Check sheet for the modelled part. Datum: model origin and axes. Units: mm. A direction names the side the tool comes from. Round coordinates to 2 decimals unless told otherwise and drop trailing zeros. Write each loop counter-clockwise with the first axis right and the second up, starting at its lowest first coordinate (ties: lowest second). Pieces come first, ordered by that corner, then holes. Notation, with made-up numbers: M -38.5,56 L 17.5,56 A27 ccw 17.5,83 Z; hole C -29,59 d1. An arc over 180 degrees is marked long. One line per item, written item: value.
from build123d import *

# Parameters (mm, degrees)
ESBO_O1_W                = 92
ESBO_O1_H                = 82
RESSALTO_EXTRUS_O1_DEPTH = 1.5
ESBO_O2_W                = 19
ESBO_O2_H                = 65
RESSALTO_EXTRUS_O2_DEPTH = 8.5
ESBO_O3_W                = 3
ESBO_O3_H                = 9
RESSALTO_EXTRUS_O3_DEPTH = 30.9
ESBO_O4_R                = 1.5
CORTE_EXTRUS_O1_DEPTH    = 3
ESBO_O5_R                = 1.5
CORTE_EXTRUS_O2_DEPTH    = 1.5
FILETE1_R                = 5
FILETE2_R                = 1


with BuildPart() as part:
    # Esboço1 → Ressalto-extrusão1 (new body)
    with BuildSketch(Plane(origin=(0, 0, 0), x_dir=(1, 0, 0), z_dir=(0, 1, 0))):
        Rectangle(ESBO_O1_W, ESBO_O1_H)
    extrude(amount=RESSALTO_EXTRUS_O1_DEPTH)

    # Esboço2 → Ressalto-extrusão2 (add)
    with BuildSketch(Plane(origin=(0, 1.5, 0), x_dir=(1, 0, 0), z_dir=(0, 1, 0))):
        with Locations((-33.5, -1.5)):
            Rectangle(ESBO_O2_W, ESBO_O2_H)
    extrude(amount=RESSALTO_EXTRUS_O2_DEPTH)

    # Esboço3 → Ressalto-extrusão3 (add)
    with BuildSketch(Plane(origin=(0, 1.5, 0), x_dir=(1, 0, 0), z_dir=(0, 1, 0))):
        with Locations((-44.5, -1.5)):
            Rectangle(ESBO_O3_W, ESBO_O3_H)
    extrude(amount=RESSALTO_EXTRUS_O3_DEPTH)

    # Esboço4 → Corte-extrusão1 (cut)
    with BuildSketch(Plane(origin=(-46, 0, 0), x_dir=(0, 0, -1), z_dir=(1, 0, 0))):
        with Locations(Location((-1.5, 30.2, 0), (0, 0, 180))):
            Circle(ESBO_O4_R)
        with Locations(Location((-1.5, 12.2, 0), (0, 0, 180))):
            Circle(ESBO_O4_R)
    extrude(amount=CORTE_EXTRUS_O1_DEPTH, mode=Mode.SUBTRACT)

    # Esboço5 → Corte-extrusão2 (cut)
    with BuildSketch(Plane(origin=(0, 1.5, 0), x_dir=(1, 0, 0), z_dir=(0, 1, 0))):
        with Locations(Location((-16.4, -1.5, 0), (0, 0, 270))):
            Circle(ESBO_O5_R)
    extrude(amount=-CORTE_EXTRUS_O2_DEPTH, mode=Mode.SUBTRACT)

    # Filete1
    filete1_edges = [part.edges().sort_by_distance(p)[0] for p in [
        (-43, 5.75, -31),
        (-43, 5.75, 34),
        (-24, 5.75, 34),
        (-24, 5.75, -31),
        (-44.5, 1.5, 6),
        (-44.5, 1.5, -3),
        (-46, 0.75, 41),
        (-46, 0.75, -41),
    ]]
    fillet(filete1_edges, radius=FILETE1_R)

    # Filete2
    filete2_edges = [part.edges().sort_by_distance(p)[0] for p in [
        (-44.5, 32.4, 6),
        (-44.5, 32.4, -3),
    ]]
    fillet(filete2_edges, radius=FILETE2_R)


solid = part.part
Q1. Sectioned sample at D-D on z = -16.5. Enter the section's corners in (x, y).
Completed:
outline: M -46,0 L 46,0 L 46,1.5 L -24,1.5 L -24,10 L -43,10 L -43,1.5 L -46,1.5 Z
Q2. Access from +Z, -Z, +X, -X, +Y, -Y to the whole of each face (thin tool, end or side, straight path). Record for faces 1 (the flat face through (-43, 6, 18)), 2 (the flat face through (-43, 21, 2)), 3 (the cylindrical face through (-26, 6, 33)).
Completed:
face 1: +Z, -X, +Y
face 2: +Z, -Z, +X, +Y
face 3: +Z, +X, +Y
Q3. Sectioned sample at A-A on z = 1.5. Enter the section's corners in (x, y), and give its area (3 significant figures).
Completed:
outline: M -46,0 L -17.9,0 L -17.9,1.5 L -24,1.5 L -24,10 L -43,10 L -43,10.7 L -46,10.7 Z; M -46,13.7 L -43,13.7 L -43,28.7 L -46,28.7 Z; M -46,31.7 L -43,31.7 L -43,32.4 L -46,32.4 Z; M -14.9,0 L 46,0 L 46,1.5 L -14.9,1.5 Z
area: 370 mm^2
Q4. Sectioned sample at C-C on y = 12.2. Enter the section's corners in (x, z), and give its area (3 significant figures).
Completed:
outline: M -46,-3 L -43,-3 L -43,0 L -46,0 Z; M -46,3 L -43,3 L -43,6 L -46,6 Z
area: 18.0 mm^2
Q5. Scan lines: line 1 (Y direction, x = -44.35, z = 1.5); line 2 (Z direction, x = -44.85, y = 30.2); line 3 (X direction, y = 0.55, z = 1.5). Record each from-to range of solid material in increasing order. Write a range as [from, to].
Completed:
line 1: [0, 10.7], [13.7, 28.7], [31.7, 32.4]
line 2: [-3, 0], [3, 6]
line 3: [-46, -17.9], [-14.9, 46]
Q6. Depth check by flat-ended pin: P1, Ø9.5, axis at y = 7, z = -17, coming from the -X side; P2, Ø7, axis at x = -32, y = 6.5, coming from the -Z side; P3, Ø3.5, axis at y = 12.2, z = 1.5, coming from the +X side; P4, Ø5, axis at x = -17, z = -25, coming from the -Y side. Enter the tip coordinate at first touch or a pass-through.
Completed:
P1: x = -43
P2: z = -31
P3: x = -43
P4: y = 0
Q7. Sectioned sample at B-B on x = -16.4. Enter the section's corners in (y, z), and give its area (4 significant figures).
Completed:
outline: M 0,-41 L 1.5,-41 L 1.5,0 L 0,0 Z; M 0,3 L 1.5,3 L 1.5,41 L 0,41 Z
area: 118.5 mm^2
